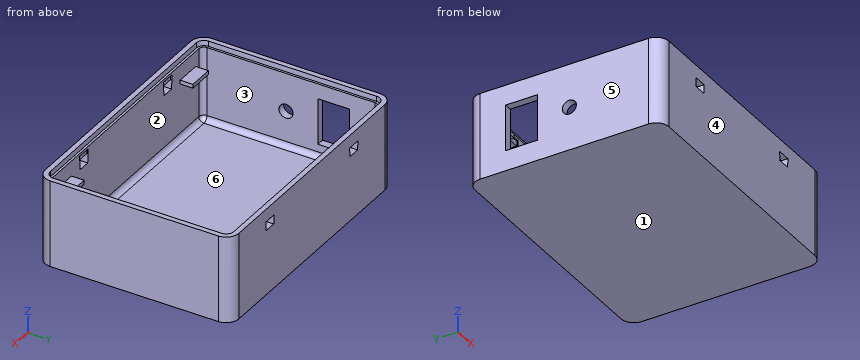
from build123d import *

# Parameters (mm, degrees)
SKETCH1_W                                = 104
SKETCH1_H                                = 76
BOSS_EXTRUDE1_DEPTH                      = 34
FILLET1_R                                = 5
SHELL1_T                                 = -3
FILLET2_R                                = 2
SKETCH2_W                                = 10
SKETCH2_H                                = 1.5
BOSS_EXTRUDE2_DEPTH                      = 5
MIRROR2_COPY_1_SKETCH_W                  = 10
MIRROR2_COPY_1_SKETCH_H                  = 1.5
MIRROR2_COPY_1_DEPTH                     = 5
LIP_GROOVE3_GROOVE_DEPTH                 = 2
LIP_GROOVE3_GROOVE_DRAFT                 = -3
SNAP_START                               = -38
SNAP_GROOVE1_DEPTH                       = 3
SNAP_START_2                             = -35.5
SNAP_GROOVE1_2_DEPTH                     = 0.5
MIRROR4_START                            = -38
MIRROR4_AT_THE_SECOND_PLANE_COPY_1_DEPTH = 3
MIRROR4_START_2                          = -35.5
MIRROR4_AT_THE_SECOND_PLANE_COPY_2_DEPTH = 0.5
MIRROR4_AT_THE_SECOND_PLANE_COPY_3_DEPTH = 0.5
SKETCH4_R                                = 2.75
SKETCH4_W                                = 18.1
SKETCH4_H                                = 12.5
CUT_EXTRUDE1_DEPTH                       = 3


# Read off the part's stored shape, not the designer's step: Lip&Groove3-Groove, Snap Groove1
with BuildPart() as part:
    # Sketch1 → Boss-Extrude1 (new body)
    with BuildSketch(Plane.XY):
        Rectangle(SKETCH1_W, SKETCH1_H)
    extrude(amount=BOSS_EXTRUDE1_DEPTH)

    # Fillet1
    fillet1_edges = [part.edges().sort_by_distance(p)[0] for p in [
        (-52, 38, 17),
        (52, 38, 17),
        (52, -38, 17),
        (-52, -38, 17),
    ]]
    fillet(fillet1_edges, radius=FILLET1_R)

    # Shell1
    shell1_openings = [part.faces().sort_by_distance(p)[0] for p in [
        (0, 0, 34),
    ]]
    offset(amount=SHELL1_T, openings=shell1_openings, kind=Kind.INTERSECTION)

    # Fillet2
    fillet2_edges = [part.edges().sort_by_distance(p)[0] for p in [
        (-49, 0, 3),
        (0, -35, 3),
        (49, 0, 3),
        (0, 35, 3),
        (-48.414213562, 34.414213562, 3),
        (48.414213562, 34.414213562, 3),
        (48.414213562, -34.414213562, 3),
        (-48.414213562, -34.414213562, 3),
    ]]
    fillet(fillet2_edges, radius=FILLET2_R)

    # Sketch2 → Boss-Extrude2 (add)
    with BuildSketch(Plane.XZ.offset(-35)):
        with Locations((-40, 25.25)):
            Rectangle(SKETCH2_W, SKETCH2_H)
    boss_extrude2 = extrude(amount=BOSS_EXTRUDE2_DEPTH)

    # Mirror1: Boss-Extrude2 across plane
    add(boss_extrude2.mirror(Plane(origin=(0, 0, 0), x_dir=(0, 0, 1), z_dir=(1, 0, 0))))

    # Mirror2: Boss-Extrude2 across plane
    add(boss_extrude2.mirror(Plane.ZX))

    # Mirror2 copy 1 sketch → Mirror2 copy 1 (add)
    with BuildSketch(Plane(origin=(0, -35, 0), x_dir=(-1, 0, 0), z_dir=(0, 1, 0))):
        with Locations((-40, 25.25)):
            Rectangle(MIRROR2_COPY_1_SKETCH_W, MIRROR2_COPY_1_SKETCH_H)
    extrude(amount=MIRROR2_COPY_1_DEPTH)


with BuildPart() as lip_groove3_groove_tool:
    # Lip&Groove3-Groove outline → Lip&Groove3-Groove (with draft: the straight prism first)
    with BuildSketch(Plane.XY.offset(32)):
        with BuildLine():
            ThreePointArc((-47, 35.895184441), (-49.047204551, 35.047204551), (-49.895184441, 33))
            Line((-49.895184441, 33), (-49.895184441, -33))
            ThreePointArc((-49.895184441, -33), (-49.047204551, -35.047204551), (-47, -35.895184441))
            Line((-47, -35.895184441), (47, -35.895184441))
            ThreePointArc((47, -35.895184441), (49.047204551, -35.047204551), (49.895184441, -33))
            Line((49.895184441, -33), (49.895184441, 33))
            ThreePointArc((49.895184441, 33), (49.047204551, 35.047204551), (47, 35.895184441))
            Line((47, 35.895184441), (-47, 35.895184441))
        make_face()
        with BuildLine():
            Line((-47, 35), (47, 35))
            ThreePointArc((47, 35), (48.414213562, 34.414213562), (49, 33))
            Line((49, 33), (49, -33))
            ThreePointArc((49, -33), (48.414213562, -34.414213562), (47, -35))
            Line((47, -35), (-47, -35))
            ThreePointArc((-47, -35), (-48.414213562, -34.414213562), (-49, -33))
            Line((-49, -33), (-49, 33))
            ThreePointArc((-49, 33), (-48.414213562, 34.414213562), (-47, 35))
        make_face(mode=Mode.SUBTRACT)
    extrude(amount=LIP_GROOVE3_GROOVE_DEPTH)
    # Lip&Groove3-Groove: the draft: its side faces are tilted about the plane it starts from
    lip_groove3_groove_sides = [lip_groove3_groove_tool.faces().sort_by_distance(p)[0] for p in [
        (-49.047204551, 35.047204551, 33),
        (-49.895184441, 0, 33),
        (-49.047204551, -35.047204551, 33),
        (0, -35.895184441, 33),
        (49.047204551, -35.047204551, 33),
        (49.895184441, 0, 33),
        (49.047204551, 35.047204551, 33),
        (0, 35.895184441, 33),
        (0, 35, 33),
        (48.414213562, 34.414213562, 33),
        (49, 0, 33),
        (48.414213562, -34.414213562, 33),
        (0, -35, 33),
        (-48.414213562, -34.414213562, 33),
        (-49, 0, 33),
        (-48.414213562, 34.414213562, 33),
    ]]
    draft(lip_groove3_groove_sides, Plane.XY.offset(32), LIP_GROOVE3_GROOVE_DRAFT)


with BuildPart() as part_1:
    add(part.part)

    # Lip&Groove3-Groove: cut by lip_groove3_groove_tool
    add(lip_groove3_groove_tool.part, mode=Mode.SUBTRACT)

    # Snap Groove1 outline → Snap Groove1 (cut)
    with BuildSketch(Plane(origin=(0, 0, 0), x_dir=(1, 0, 0), z_dir=(0, 1, 0)).offset(SNAP_START)):
        Polygon((-29.47379611, -25.5), (-29.657223337, -29), (-24.342776662, -29), (-24.52620389, -25.5), align=None)
    snap_groove1 = extrude(amount=SNAP_GROOVE1_DEPTH, mode=Mode.SUBTRACT)

    # Snap Groove1 2 outline → Snap Groove1 2 (cut)
    with BuildSketch(Plane(origin=(0, 0, 0), x_dir=(1, 0, 0), z_dir=(0, 1, 0)).offset(SNAP_START_2)):
        Polygon((-24.342776662, -29), (-29.657223338, -29), (-29.762038896, -31), (-24.237961104, -31), align=None)
    snap_groove1_2 = extrude(amount=SNAP_GROOVE1_2_DEPTH, mode=Mode.SUBTRACT)

    # Mirror4: Snap Groove1, Snap Groove1 2 across plane
    add(snap_groove1.mirror(Plane(origin=(0, 0, 0), x_dir=(0, 0, 1), z_dir=(1, 0, 0))), mode=Mode.SUBTRACT)
    add(snap_groove1_2.mirror(Plane(origin=(0, 0, 0), x_dir=(0, 0, 1), z_dir=(1, 0, 0))), mode=Mode.SUBTRACT)

    # Mirror4 at the second plane: Snap Groove1, Snap Groove1 2 across plane
    add(snap_groove1.mirror(Plane.ZX), mode=Mode.SUBTRACT)
    add(snap_groove1_2.mirror(Plane.ZX), mode=Mode.SUBTRACT)

    # Mirror4 at the second plane copy 1 sketc → Mirror4 at the second plane copy 1 (cut)
    with BuildSketch(Plane(origin=(0, 0, 0), x_dir=(-1, 0, 0), z_dir=(0, -1, 0)).offset(MIRROR4_START)):
        Polygon((-29.47379611, -25.5), (-29.657223337, -29), (-24.342776662, -29), (-24.52620389, -25.5), align=None)
    extrude(amount=MIRROR4_AT_THE_SECOND_PLANE_COPY_1_DEPTH, mode=Mode.SUBTRACT)

    # Mirror4 at the second plane copy 2 sketc → Mirror4 at the second plane copy 2 (cut)
    with BuildSketch(Plane(origin=(0, 0, 0), x_dir=(-1, 0, 0), z_dir=(0, -1, 0)).offset(MIRROR4_START_2)):
        Polygon((-24.342776662, -29), (-29.657223338, -29), (-29.762038896, -31), (-24.237961104, -31), align=None)
    extrude(amount=MIRROR4_AT_THE_SECOND_PLANE_COPY_2_DEPTH, mode=Mode.SUBTRACT)

    # Mirror4 at the second plane copy 3 sketc → Mirror4 at the second plane copy 3 (cut)
    with BuildSketch(Plane.XZ.offset(MIRROR4_START_2)):
        Polygon((-24.342776662, 29), (-29.657223338, 29), (-29.762038896, 31), (-24.237961104, 31), align=None)
    extrude(amount=MIRROR4_AT_THE_SECOND_PLANE_COPY_3_DEPTH, mode=Mode.SUBTRACT)

    # Sketch4 → Cut-Extrude1 (cut)
    with BuildSketch(Plane.ZY.offset(52)):
        with Locations(Location((17, -2, 0), (0, 0, 270))):
            Circle(SKETCH4_R)
        with Locations((17.05, 16.75)):
            Rectangle(SKETCH4_W, SKETCH4_H)
    extrude(amount=-CUT_EXTRUDE1_DEPTH, mode=Mode.SUBTRACT)


solid = part_1.part
Here's how the part is built. I have some questions about the finished solid (model axes, mm). Face numbers are marked on the shaded views. A direction names the side the tool comes from. Coordinates: 2 decimals unless noted, no trailing zeros. Loops run counter-clockwise (first coordinate to the right, second up) from the corner with the lowest first, then second, coordinate; pieces in that order, holes last. Notation, with made-up numbers: (8.5, 73.25) -> (18.5, 73.25) arc R16 cw to (18.5, 93.25) -> close; hole circle Ø4 at (12.25, 80). An arc over 180 degrees is marked (long way). Use one line per item in the form item = value. Start each with the question number.
(1) We'd pull the mould along X, two halves only. Please class the marked faces 3, 4, 5 and 6: pulls with the +X half, pulls with the -X half, needs draft (parallel to the pull), parting line crosses it, or undercut.
(2) If we section it at D-D (x = 41): Please give me the cut outline in (y, z), then the cut area to 3 significant figures.
(3) If we section it at C-C (x = -15): Please give me the cut outline in (y, z), then the cut area to 3 significant figures.
(4) If we section it at A-A (y = -2): Please give me the cut outline in (x, z), then the cut area to 3 significant figures.
(5) On a 3-axis mill with a long thin cutter (end or side, diameter ignored), from which of +Z, -Z, +X, -X, +Y, -Y can I reach the whole of each face in a straight line? I mean the marked faces 1 and 2. Say none if no direction works.
(6) Will these pins go through, and if not, where does the flat tip stop? pin 1 (4 mm diameter, centred on x = -38.5, y = -33.5, fed in from +Z); pin 2 (1.5 mm diameter, centred on x = -20, y = 23, fed in from +Z); pin 3 (1 mm diameter, centred on y = 21, z = 23.5, fed in from -X).
(7) Please list where these lines run through material, in increasing order: line 1 along Y through (x, z) = (-11, 23); line 2 along X through (y, z) = (-29, 14.5); line 3 along Y through (x, z) = (37.5, 25).
(8) If we section it at B-B (z = 17): Please give me the cut outline in (x, y), then the cut area to 3 significant figures.
Verdict:
q1.face_3 = undercut
q1.face_4 = needs draft
q1.face_5 = pulls with the -X half
q1.face_6 = undercut
q2.outline = (-38, 0) -> (38, 0) -> (38, 34) -> (36, 34) -> (35.9, 32) -> (35, 32) -> (35, 26) -> (30, 26) -> (30, 24.5) -> (35, 24.5) -> (35, 5) arc R2 cw to (33, 3) -> (-33, 3) arc R2 cw to (-35, 5) -> (-35, 24.5) -> (-30, 24.5) -> (-30, 26) -> (-35, 26) -> (-35, 32) -> (-35.9, 32) -> (-36, 34) -> (-38, 34) -> close
q2.area = 427 mm²
q3.outline = (-38, 0) -> (38, 0) -> (38, 34) -> (36, 34) -> (35.9, 32) -> (35, 32) -> (35, 5) arc R2 cw to (33, 3) -> (-33, 3) arc R2 cw to (-35, 5) -> (-35, 32) -> (-35.9, 32) -> (-36, 34) -> (-38, 34) -> close
q3.area = 412 mm²
q4.outline = (-52, 0) -> (52, 0) -> (52, 34) -> (50, 34) -> (49.9, 32) -> (49, 32) -> (49, 5) arc R2 cw to (47, 3) -> (-47, 3) arc R2 cw to (-49, 5) -> (-49, 14.25) -> (-52, 14.25) -> close; (-52, 19.75) -> (-49, 19.75) -> (-49, 32) -> (-49.9, 32) -> (-50, 34) -> (-52, 34) -> close
q4.area = 479 mm²
q5.face_1 = -Z, +X, -X, +Y, -Y
q5.face_2 = none
q6.pin_1 = 32
q6.pin_2 = 3
q6.pin_3 = 49
q7.line_1 = -38 to -35, 35 to 38
q7.line_2 = -52 to -49, 49 to 52
q7.line_3 = -38 to -30, 30 to 38
q8.outline = (-52, -33) arc R5 ccw to (-47, -38) -> (47, -38) arc R5 ccw to (52, -33) -> (52, 33) arc R5 ccw to (47, 38) -> (-47, 38) arc R5 ccw to (-52, 33) -> (-52, 23) -> (-49, 23) -> (-49, 33) arc R2 cw to (-47, 35) -> (47, 35) arc R2 cw to (49, 33) -> (49, -33) arc R2 cw to (47, -35) -> (-47, -35) arc R2 cw to (-49, -33) -> (-49, -4.75) -> (-52, -4.75) -> close; (-52, 0.75) -> (-49, 0.75) -> (-49, 10.5) -> (-52, 10.5) -> close
q8.area = 972 mm²
